```python
from build123d import *

# Parameters (mm, degrees)
SKETCH_R           = 11
PAD_DEPTH          = 2
SKETCH001_R        = 11
SKETCH002_R        = 8
FILLET_R           = 7
SKETCH003_R        = 1.75
POCKET_DEPTH       = 12.001
SKETCH004_R        = 4
POCKET001_DEPTH    = 9
FILLET001_R        = 1
FILLET002_R        = 1
POCKET002_DEPTH    = 2
POLARPATTERN_COUNT = 6


with BuildPart() as part:
    # Sketch → Pad (new body)
    with BuildSketch(Plane.XY):
        Circle(SKETCH_R)
    extrude(amount=PAD_DEPTH)

    # Sketch001 (on Face3 of Pad) → AdditiveLoft section 0
    with BuildSketch(Plane.XY.offset(2)):
        Circle(SKETCH001_R)
    # Sketch002 (on DatumPlane) → AdditiveLoft section 1
    with BuildSketch(Plane.XY.offset(12)):
        Circle(SKETCH002_R)
    loft()

    # Fillet
    fillet_edges = [part.edges().sort_by_distance(p)[0] for p in [
        (-11, 0, 2),
    ]]
    fillet(fillet_edges, radius=FILLET_R)

    # Sketch003 (on Face5 of Fillet) → Pocket (cut, through all)
    with BuildSketch(Plane.XY.offset(12)):
        Circle(SKETCH003_R)
    extrude(amount=-POCKET_DEPTH, mode=Mode.SUBTRACT)

    # Sketch004 (on Face6 of Pocket) → Pocket001 (cut)
    with BuildSketch(Plane.XY.offset(12)):
        Circle(SKETCH004_R)
    extrude(amount=-POCKET001_DEPTH, mode=Mode.SUBTRACT)

    # Fillet001
    fillet001_edges = [part.edges().sort_by_distance(p)[0] for p in [
        (-8, 0, 12),
    ]]
    fillet(fillet001_edges, radius=FILLET001_R)

    # Fillet002
    fillet002_edges = [part.edges().sort_by_distance(p)[0] for p in [
        (-4, 0, 12),
    ]]
    fillet(fillet002_edges, radius=FILLET002_R)

    # Sketch005 (on Face1 of Fillet002) → Pocket002 (cut)
    with BuildSketch(Plane.XY.offset(12)):
        with BuildLine():
            Line((-9.659258, 2.58819), (-4.829629, 1.294095))
            Line((-4.829629, 1.294095), (-1.931852, 0.517638))
            ThreePointArc((-1.931852, 0.517638), (-2, 0), (-1.931852, -0.517638))
            Line((-4.829629, -1.294095), (-1.931852, -0.517638))
            Line((-9.659258, -2.58819), (-4.829629, -1.294095))
            ThreePointArc((-9.659258, 2.58819), (-10, 0), (-9.659258, -2.58819))
        make_face()
    pocket002 = extrude(amount=-POCKET002_DEPTH, mode=Mode.SUBTRACT)

    # PolarPattern: Pocket002 ×6 about axis
    polarpattern_axis = Axis((0, 0, 12), (0, 0, 1))
    for i in range(1, POLARPATTERN_COUNT):
        add(pocket002.rotate(polarpattern_axis, i * 360 / POLARPATTERN_COUNT), mode=Mode.SUBTRACT)


solid = part.part
```
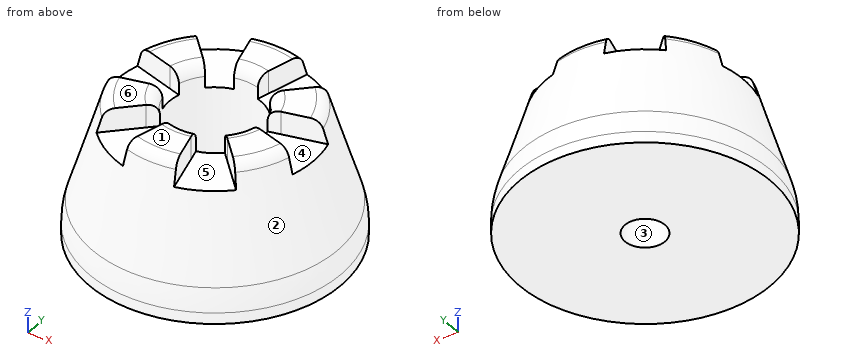
Geometry check sheet. Reference: the model listing, model coordinates, mm. Face numbers are marked on the shaded views. A direction names the side the tool comes from. Round coordinates to 2 decimals unless told otherwise and drop trailing zeros. Loops run counter-clockwise (first coordinate to the right, second up) from the corner with the lowest first, then second, coordinate; pieces in that order, holes last. Notation, with made-up numbers: M 53,3.5 L 104,3.5 A21 cw 104,31.5 Z; hole C -6,72 d5. An arc over 180 degrees is marked long. Return JSON: item names as keys, results as strings. Group by question number.
(1) Mould release check, pull along Y, two halves, no side actions. Record for the marked faces 1, 2 and 3: pulls with the +Y half, pulls with the -Y half, needs draft (parallel to the pull), parting line crosses it, or undercut.
(2) Section check A-A, the plane z = 4. Enter the section's corners in (x, y).
(3) Set-up check for the marked faces 4, 5 and 6: record each of +Z, -Z, +X, -X, +Y, -Y from which the full face is reachable in a straight line by a thin tool's end or side.
(4) Scan lines: line 1 along Y through (x, z) = (0, 0.9); line 2 along Z through (x, y) = (-5.5, 0.25); line 3 along Y through (x, z) = (0, 8.5). Record each from-to range of solid material in increasing order. Write a range as [from, to].
(5) Go/stop test with flat-tipped pins: pin 1 (2 mm diameter, centred on y = -8, z = 2, fed in from -X); pin 2 (2.5 mm diameter, centred on x = -4.5, y = 6.5, fed in from +Z); pin 3 (4 mm diameter, centred on y = -1, z = 9, fed in from +X). Record where each tip stops, or that it passes through.
Data:
{
 "1": {"face 1": "needs draft", "face 2": "parting line crosses it", "face 3": "undercut"},
 "2": {"outline": "C 0,0 d20.8; hole C 0,0 d8"},
 "3": {"face 4": "+Z, +X", "face 5": "+Z", "face 6": "+Z, +X, -X, +Y, -Y"},
 "4": {"line 1": "[-11, -1.75], [1.75, 11]", "line 2": "[0, 10]", "line 3": "[-9.05, -4], [4, 9.05]"},
 "5": {"pin 1": "x = -8.4", "pin 2": "z = 10", "pin 3": "x = 9.47"}
}
